The listing builds one solid part. Answer for the finished solid, in the listing's coordinates (mm). Give positions to 0.01 mm unless a question says otherwise; leave off trailing zeros. Write each loop counter-clockwise with the first axis right and the second up, starting at its lowest first coordinate (ties: lowest second). Pieces come first, ordered by that corner, then holes. Notation, with made-up numbers: (19, 57) -> (30, 57) arc R14 ccw to (30, 78) -> close; hole circle Ø2 at (3.25, -39.75). An arc over 180 degrees is marked (long way). Put each result on its own line as item: value. Start each with the question number.
1) For a pull along X with two mould halves and no side action, classify faces 1 (the cylindrical face through (53.025, -3.857, 3.913)), 2 (the cylindrical face through (42.11, -3.21, 3.91)), 3 (the cylindrical face through (-3.968, -3.881, 3.913)), 4 (the flat face through (39, -1, 0)) as released by +X, released by -X, zero draft, split by the parting line, or undercut.
2) Flat-ended cylindrical pins translate along their axes: pin 1 Ø2 at (x, z) = (29.5, 5.5) entering from +Y; pin 2 Ø1.5 at (y, z) = (-5.5, 5.5) entering from +X. Find the tip coordinate at first contact, or state that the pin passes through.
3) A cutting plane is placed at A-A (x = 63.5). Write down the section's boundary in (y, z), then the cut area to 3 significant figures.
4) A cutting plane is placed at B-B (z = 4.25). Give the number of separate pieces and of enclosed holes in the cut face, then the cut area to 3 significant figures.
5) A cutting plane is placed at C-C (x = 17). Write down the section's boundary in (y, z), then the cut area to 3 significant figures.
6) Find the intervals of material crossed by line 1 along Y through (x, z) = (31.75, 4.5); line 2 along Y through (x, z) = (56, 4); line 3 along X through (y, z) = (-7.25, 1.25), in increasing order. Write a range as from..to.
from build123d import *

# Parameters (mm, degrees)
F0_R     = 2.54
F1_DEPTH = 7.9375


with BuildPart() as f1:
    # F0 (on Top) → F1 (new body)
    with BuildSketch(Plane.XY):
        with BuildLine():
            Line((79.375, 0), (0, 0))
            Line((0, 0), (0, -1.42875))
            ThreePointArc((0, -1.42875), (1.796051, -2.172699), (2.54, -3.96875))
            ThreePointArc((2.54, -3.96875), (1.796051, -5.764801), (0, -6.50875))
            Line((0, -6.50875), (0, -7.9375))
            Line((0, -7.9375), (79.375, -7.9375))
            ThreePointArc((79.375, -7.9375), (83.34375, -3.96875), (79.375, 0))
        make_face()
        with Locations((7.9375, -3.96875)):
            Circle(F0_R, mode=Mode.SUBTRACT)
        with Locations((15.875, -3.96875)):
            Circle(F0_R, mode=Mode.SUBTRACT)
        with Locations((23.8125, -3.96875)):
            Circle(F0_R, mode=Mode.SUBTRACT)
        with Locations((31.75, -3.96875)):
            Circle(F0_R, mode=Mode.SUBTRACT)
        with Locations((39.6875, -3.96875)):
            Circle(F0_R, mode=Mode.SUBTRACT)
        with Locations((47.625, -3.96875)):
            Circle(F0_R, mode=Mode.SUBTRACT)
        with Locations((55.5625, -3.96875)):
            Circle(F0_R, mode=Mode.SUBTRACT)
        with Locations((63.5, -3.96875)):
            Circle(F0_R, mode=Mode.SUBTRACT)
        with Locations((71.4375, -3.96875)):
            Circle(F0_R, mode=Mode.SUBTRACT)
        with Locations((79.375, -3.96875)):
            Circle(F0_R, mode=Mode.SUBTRACT)
        with BuildLine():
            Line((0, -1.42875), (0, 0))
            ThreePointArc((0, 0), (-3.96875, -3.96875), (0, -7.9375))
            Line((0, -7.9375), (0, -6.50875))
            ThreePointArc((0, -6.50875), (-2.54, -3.96875), (0, -1.42875))
        make_face()
    extrude(amount=F1_DEPTH)


solid = f1.part
Reply:
1. face 1: undercut
1. face 2: undercut
1. face 3: released by -X
1. face 4: zero draft
2. pin 1: stops at y = 0
2. pin 2: stops at x = 83.27
3. outline: (-7.94, 0) -> (-6.51, 0) -> (-6.51, 7.94) -> (-7.94, 7.94) -> close; (-1.43, 0) -> (0, 0) -> (0, 7.94) -> (-1.43, 7.94) -> close
3. area: 22.7 mm2
4. separate pieces: 1
4. enclosed holes: 11
4. area: 457 mm2
5. outline: (-7.94, 0) -> (-6.25, 0) -> (-6.25, 7.94) -> (-7.94, 7.94) -> close; (-1.69, 0) -> (0, 0) -> (0, 7.94) -> (-1.69, 7.94) -> close
5. area: 26.9 mm2
6. line 1: y = -7.94..-6.51, -1.43..0
6. line 2: y = -7.94..-6.47, -1.47..0
6. line 3: x = -2.23..81.61
